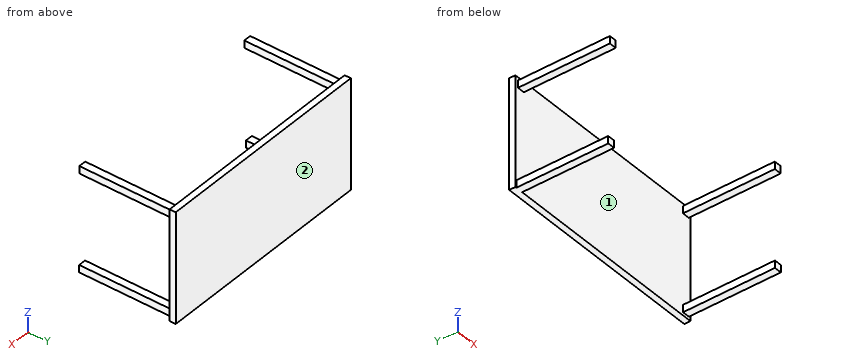
from build123d import *

# Parameters (mm, degrees)
SKETCH_W     = 1800
SKETCH_H     = 900
PAD_DEPTH    = 50
SKETCH001_W  = 60
SKETCH001_H  = 60
PAD001_DEPTH = 750


with BuildPart() as part:
    # Sketch → Pad (new body)
    with BuildSketch(Plane.XZ):
        with Locations((900, 450)):
            Rectangle(SKETCH_W, SKETCH_H)
    extrude(amount=PAD_DEPTH)

    # Sketch001 (on Face6 of Pad) → Pad001 (join)
    with BuildSketch(Plane.XZ.offset(50)):
        with Locations((1755.017945, 55.870171)):
            Rectangle(SKETCH001_W, SKETCH001_H)
        with Locations((1753.631055, 851.470837)):
            Rectangle(SKETCH001_W, SKETCH001_H)
        with Locations((40.092932, 30)):
            Rectangle(SKETCH001_W, SKETCH001_H)
        with Locations((57.324378, 845.378981)):
            Rectangle(SKETCH001_W, SKETCH001_H)
    extrude(amount=PAD001_DEPTH)


solid = part.part
Could you check a few things on this model? Use its own coordinates, in mm. Face numbers are marked on the shaded views. Give positions to 0.01 mm unless a question says otherwise; leave off trailing zeros. Write each loop counter-clockwise with the first axis right and the second up, starting at its lowest first coordinate (ties: lowest second). Pieces come first, ordered by that corner, then holes. Notation, with made-up numbers: (29.5, 36) -> (68.5, 36) arc R20 ccw to (68.5, 45) -> close; hole circle Ø11 at (88.25, 40). An arc over 180 degrees is marked (long way). Answer as CSV lines item,"result". Start each with the question number.
(1) If we section it at A-A, the plane y = -331: Write out the boundary of the cut face in (x, z), and give its area (3 significant figures).
(2) If we section it at C-C, the plane x = 1608: Write out the boundary of the cut face in (y, z), and give its area (3 significant figures).
(3) Please list where these lines run through material, in increasing order: line 1 (X direction, y = -72, z = 852); line 2 (Y direction, x = 1044.5, z = 227); line 3 (X direction, y = -633, z = 82).
(4) If we section it at B-B, the plane z = 207: Write out the boundary of the cut face in (x, y), and give its area (3 significant figures).
(5) I'm going to push flat-ended pins straight in: pin 1 Ø18 at (y, z) = (-548, 43.5) entering from -X; pin 2 Ø18 at (x, y) = (1744.5, -294) entering from +Z; pin 3 Ø18 at (y, z) = (-542.5, 846) entering from -X. Where does each tip first touch, or does it pass through?
(6) If we mould it in two halves opening along X, with no side actions, what happens to the marked faces 1 and 2? For each: +X half, -X half, draft (parallel to the pull), parting line (faces both ways), or undercut.
Answer list:
1,outline,"(10.09, 0) -> (70.09, 0) -> (70.09, 60) -> (10.09, 60) -> close; (27.32, 815.38) -> (87.32, 815.38) -> (87.32, 875.38) -> (27.32, 875.38) -> close; (1723.63, 821.47) -> (1783.63, 821.47) -> (1783.63, 881.47) -> (1723.63, 881.47) -> close; (1725.02, 25.87) -> (1785.02, 25.87) -> (1785.02, 85.87) -> (1725.02, 85.87) -> close"
1,area,"14,400 mm^2"
2,outline,"(-50, 0) -> (0, 0) -> (0, 900) -> (-50, 900) -> close"
2,area,"45,000 mm^2"
3,line 1,"27.32 to 87.32, 1723.63 to 1783.63"
3,line 2,"-50 to 0"
3,line 3,"1725.02 to 1785.02"
4,outline,"(0, -50) -> (1800, -50) -> (1800, 0) -> (0, 0) -> close"
4,area,"90,000 mm^2"
5,pin 1,"x = 10.09"
5,pin 2,"z = 881.47"
5,pin 3,"x = 27.32"
6,face 1,"undercut"
6,face 2,"draft"
